Model file for the job. Use its own axes, mm. Face numbers are marked on the shaded views. A direction names the side the tool comes from. Coordinates: 2 decimals unless noted, no trailing zeros. Order: outer loops, then holes, each group sorted by start corner. A loop starts at its lowest first (then second) coordinate and runs counter-clockwise, first axis right, second up. Notation, with made-up numbers: (-8, -5) -> (0, -5) arc R19 cw to (0, 17) -> close; hole circle Ø4 at (7, -28.5). An arc over 180 degrees is marked (long way). Return JSON: item names as keys, results as strings. Group by question number.
1) Cut at B-B (z = -16.5). Write the cut outline in (x, y), and give its area (3 significant figures).
2) Flat gauge pins, fed straight in: pin 1 (1.4 mm diameter, centred on x = 22.5, y = -1.5, fed in from -Z); pin 2 (2.5 mm diameter, centred on y = -1, z = -11.5, fed in from -X); pin 3 (0.9 mm diameter, centred on y = -2, z = -23.5, fed in from -X); pin 4 (1.6 mm diameter, centred on y = -19.36, z = -38.95, fed in from -X). Where does each tip first touch, or does it go through?
3) Probe line 1 (X direction, y = -39, z = -6.5); line 2 (Z direction, x = -51.7, y = -15.85); line 3 (Y direction, x = 2, z = -17). List the from-to ranges inside material, lowest first.
4) Which spindle directions (+Z, -Z, +X, -X, +Y, -Y) get a long thin tool onto all of the face, cutting with end or side? Do the marked faces 1 and 2. Say none if no direction does.
5) Cut at A-A (y = -22). Write the cut outline in (x, z).
6) Pull direction X, two halves, no side cores. Call the marked faces 3, 4, 5 and 6: +X half, -X half, draft (parallel to the pull), parting line (faces both ways), or undercut.
7) Cut at C-C (x = 11). Write the cut outline in (y, z), and give its area (3 significant figures).
from build123d import *

# Parameters (mm, degrees)
SKETCH1_W               = 2.9
SKETCH1_H               = 5
SKETCH1_W_2             = 6
BASE_FLANGE1_DEPTH      = 3
SKETCHED_START          = -41.587720567
SKETCHED_BEND1_DEPTH    = 54.641148945
SKETCHED_BEND1_2_DEPTH  = 9.641148945
SKETCHED_BEND1_3_DEPTH  = 54.641148945
SKETCHED_START_2        = -31.946571622
SKETCHED_BEND1_4_DEPTH  = 45
CUT_EXTRUDE2_DEPTH      = 122.204531689
CUT_EXTRUDE2_DEPTH_BACK = 122.204531689
SKETCH32_R              = 1


# Read off the part's stored shape, not the designer's step: Sketched Bend1
# Sheet-metal steps are written as plain solids
with BuildPart() as part:
    # Sketch1 → Base-Flange1 (new body)
    with BuildSketch(Plane(origin=(0, 0, 0), x_dir=(1, 0, 0), z_dir=(0, 1, 0))):
        Polygon((-80, 31.946571622), (-80, -13.053428378), (80, -13.053428378), (80, 31.946571622), (80, 41.587720567), (45, 41.587720567), (45, 31.946571622), (-45, 31.946571622), (-45, 41.587720567), (-80, 41.587720567), align=None)
        with Locations((-39.45, 10.905641405)):
            Rectangle(SKETCH1_W, SKETCH1_H, mode=Mode.SUBTRACT)
        with Locations((-22.55, 22.947848405)):
            Rectangle(SKETCH1_W, SKETCH1_H, mode=Mode.SUBTRACT)
        with Locations((-31, 22.946571622)):
            Rectangle(SKETCH1_W_2, SKETCH1_H, mode=Mode.SUBTRACT)
        with Locations((-31, 10.946571622)):
            Rectangle(SKETCH1_W_2, SKETCH1_H, mode=Mode.SUBTRACT)
        with Locations((31, 10.946571622)):
            Rectangle(SKETCH1_W_2, SKETCH1_H, mode=Mode.SUBTRACT)
        with Locations((31, 22.946571622)):
            Rectangle(SKETCH1_W_2, SKETCH1_H, mode=Mode.SUBTRACT)
        with Locations((22.55, 22.947848405)):
            Rectangle(SKETCH1_W, SKETCH1_H, mode=Mode.SUBTRACT)
        with Locations((39.45, 10.905641405)):
            Rectangle(SKETCH1_W, SKETCH1_H, mode=Mode.SUBTRACT)
    extrude(amount=-BASE_FLANGE1_DEPTH)

    # Sketched Bend1 outline → Sketched Bend1 (cut)
    with BuildSketch(Plane.XY.offset(SKETCHED_START)):
        with BuildLine():
            Line((50.848469227, -3), (80, -3))
            Line((80, -3), (80, 0))
            Line((80, 0), (43.5, 0))
            ThreePointArc((43.5, 0), (47.468626966, -0.778888953), (50.848469227, -3))
        make_face()
        with BuildLine():
            Line((-43.5, 0), (-80, 0))
            Line((-80, 0), (-80, -3))
            Line((-80, -3), (-50.848469227, -3))
            ThreePointArc((-50.848469227, -3), (-47.468626966, -0.778888953), (-43.5, 0))
        make_face()
    extrude(amount=SKETCHED_BEND1_DEPTH, mode=Mode.SUBTRACT)

    # Sketched Bend1 2 outline → Sketched Bend1 2 (cut)
    with BuildSketch(Plane.XY.offset(SKETCHED_START)):
        with BuildLine():
            Line((45, -3), (50.848469227, -3))
            ThreePointArc((50.848469227, -3), (48.154590073, -1.088050614), (45, -0.107695155))
            Line((45, -0.107695155), (45, -3))
        make_face()
        with BuildLine():
            Line((-50.848469227, -3), (-45, -3))
            Line((-45, -3), (-45, -0.107695155))
            ThreePointArc((-45, -0.107695155), (-48.154590073, -1.088050614), (-50.848469227, -3))
        make_face()
    extrude(amount=SKETCHED_BEND1_2_DEPTH, mode=Mode.SUBTRACT)



with BuildPart() as body_2:
    # Sketched Bend1 3 outline → Sketched Bend1 3 (new body)
    with BuildSketch(Plane.XY.offset(SKETCHED_START)):
        with BuildLine():
            Line((50.924621202, -3.075378798), (48.803300859, -5.196699141))
            ThreePointArc((48.803300859, -5.196699141), (50.429096494, -7.629874257), (51, -10.5))
            Line((51, -10.5), (51, -44))
            Line((51, -44), (54, -44))
            Line((54, -44), (54, -10.5))
            ThreePointArc((54, -10.5), (53.200735091, -6.48182396), (50.924621202, -3.075378798))
        make_face()
        with BuildLine():
            ThreePointArc((-51, -10.5), (-50.429096494, -7.629874257), (-48.803300859, -5.196699141))
            Line((-48.803300859, -5.196699141), (-50.924621202, -3.075378798))
            ThreePointArc((-50.924621202, -3.075378798), (-53.200735091, -6.48182396), (-54, -10.5))
            Line((-54, -10.5), (-54, -44))
            Line((-54, -44), (-51, -44))
            Line((-51, -44), (-51, -10.5))
        make_face()
    extrude(amount=SKETCHED_BEND1_3_DEPTH)


with BuildPart() as part_1:
    add(part.part)

    add(body_2.part)  # Sketched Bend1 4 merges body 2
    # Sketched Bend1 4 outline → Sketched Bend1 4 (add)
    with BuildSketch(Plane.XY.offset(SKETCHED_START_2)):
        with BuildLine():
            ThreePointArc((43.5, -3), (46.370125743, -3.570903506), (48.803300859, -5.196699141))
            Line((48.803300859, -5.196699141), (50.924621202, -3.075378798))
            ThreePointArc((50.924621202, -3.075378798), (50.886641368, -3.037592259), (50.848469227, -3))
            Line((50.848469227, -3), (43.5, -3))
        make_face()
        with BuildLine():
            ThreePointArc((-48.803300859, -5.196699141), (-46.370125743, -3.570903506), (-43.5, -3))
            Line((-43.5, -3), (-50.848469227, -3))
            ThreePointArc((-50.848469227, -3), (-50.886641368, -3.037592259), (-50.924621202, -3.075378798))
            Line((-50.924621202, -3.075378798), (-48.803300859, -5.196699141))
        make_face()
    extrude(amount=SKETCHED_BEND1_4_DEPTH)

    # Sketch32 → Cut-Extrude2 (cut, two sides: drawn at the far end of the back side and taken through both)
    with BuildSketch(Plane.ZY.offset(-51).offset(-CUT_EXTRUDE2_DEPTH_BACK)):
        with Locations(Location((-38.946571622, -19.363015099, 0), (0, 0, 270))):
            Circle(SKETCH32_R)
        with Locations(Location((-38.946571622, -15.85, 0), (0, 0, 270))):
            Circle(SKETCH32_R)
    extrude(amount=CUT_EXTRUDE2_DEPTH + CUT_EXTRUDE2_DEPTH_BACK, mode=Mode.SUBTRACT)


solid = part_1.part
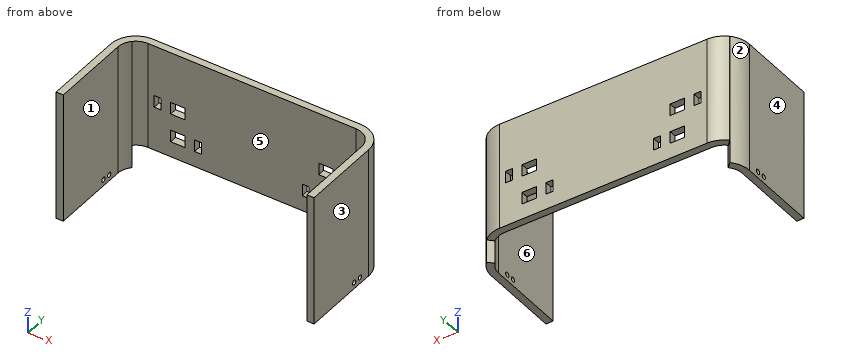
Answers below:
{
 "1": {"outline": "(-54, -44) -> (-51, -44) -> (-51, -10.5) arc R7.5 cw to (-43.5, -3) -> (43.5, -3) arc R7.5 cw to (51, -10.5) -> (51, -44) -> (54, -44) -> (54, -10.5) arc R10.5 ccw to (50.92, -3.08) arc R10.5 ccw to (50.85, -3) arc R10.5 ccw to (43.5, 0) -> (-43.5, 0) arc R10.5 ccw to (-50.85, -3) arc R10.5 ccw to (-50.92, -3.08) arc R10.5 ccw to (-54, -10.5) -> close", "area": "547 mm^2"},
 "2": {"pin 1": "stops at z = -31.95", "pin 2": "stops at x = -50", "pin 3": "stops at x = -50.24", "pin 4": "passes through"},
 "3": {"line 1": "x = -54 to -51, 51 to 54", "line 2": "z = -41.59 to -39.95, -37.95 to 13.05", "line 3": "y = -3 to 0"},
 "4": {"face 1": "+Z, -Z, -Y", "face 2": "+Z, -Z, -X, +Y"},
 "5": {"outline": "(-54, -41.59) -> (-51, -41.59) -> (-51, 13.05) -> (-54, 13.05) -> close; (51, -41.59) -> (54, -41.59) -> (54, 13.05) -> (51, 13.05) -> close"},
 "6": {"face 3": "+X half", "face 4": "-X half", "face 5": "undercut", "face 6": "undercut"},
 "7": {"outline": "(-3, -31.95) -> (0, -31.95) -> (0, 13.05) -> (-3, 13.05) -> close", "area": "135 mm^2"}
}
